Read the model definition and answer for the solid it produces. Units are mm, in the model's axes. Face numbers are marked on the shaded views. A direction names the side the tool comes from. Coordinates: 2 decimals unless noted, no trailing zeros. Write each loop counter-clockwise with the first axis right and the second up, starting at its lowest first coordinate (ties: lowest second). Pieces come first, ordered by that corner, then holes.
(1) Given pin 1 (1.5 mm diameter, centred on x = -4.5, y = 2, fed in from +Z); pin 2 (10.5 mm diameter, centred on x = 0, y = -3, fed in from +Z); pin 3 (1.5 mm diameter, centred on y = 7.5, z = 14.5, fed in from -X); pin 4 (3.5 mm diameter, centred on x = 0, y = 0, fed in from +Z), each flat-ended and moving along its own axis, determine where each tip first touches the part or whether it passes through.
(2) Which of the six approach directions +Z, -Z, +X, -X, +Y, -Y give full straight-line access (tool end or side, diameter ignored) to the marked faces 4 and 5?
(3) Find the intervals of material crossed by probe 1 along Y at (x, z) = (0, 3.55) (3 decimals); probe 2 along Y at (x, z) = (0, 8.45) (3 decimals); probe 3 along Z at (x, y) = (-6, 1.5), in increasing order.
(4) The mould has two halves that part along X. Classify the marked faces 1, 2 and 3: +X half, -X half, draft (parallel to the pull), parting line (faces both ways), or undercut.
(5) Section D-D on z = 10.5 is taken. Write down the section's boundary in (x, y) (3 decimals).
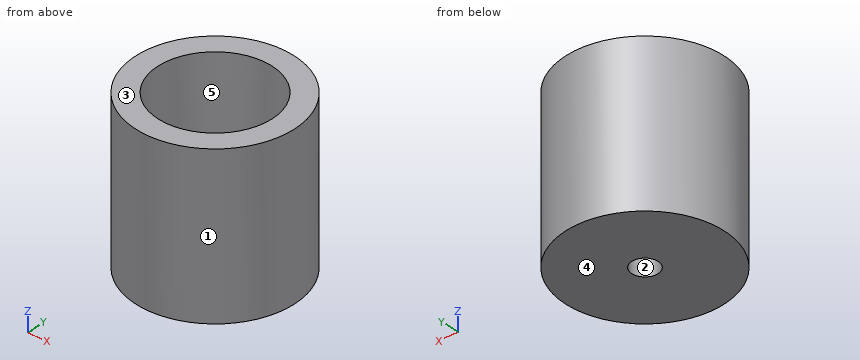
from build123d import *

# Parameters (mm, degrees)
SKETCH1_R                                        = 9.525
BOSS_EXTRUDE1_DEPTH                              = 19.05
CBORE_FOR_1_4_SOCKET_HEAD_CAP_SCREW1_D           = 0.79375
CBORE_FOR_1_4_SOCKET_HEAD_CAP_SCREW1_DEPTH       = 12.7
CBORE_FOR_1_4_SOCKET_HEAD_CAP_SCREW1_CBORE_D     = 3.175
CBORE_FOR_1_4_SOCKET_HEAD_CAP_SCREW1_CBORE_DEPTH = 3.175
CBORE_FOR_1_4_SOCKET_HEAD_CAP_SCREW1_TIP         = 0.238466558


with BuildPart() as part:
    # Sketch1 → Boss-Extrude1 (new body)
    with BuildSketch(Plane.XY):
        Circle(SKETCH1_R)
    extrude(amount=BOSS_EXTRUDE1_DEPTH)

    # Sketch6 → 1/4 NPT Tapped Hole1 (revolve, cut)
    with BuildSketch(Plane(origin=(0, 0, 19.05), x_dir=(0, -1, 0), z_dir=(1, 0, 0))):
        Polygon((0, 0), (0, 14.772347279), (5.5626, 11.43), (5.5626, 10.0203), (6.557978799, 10.0203), (6.858, 0), align=None)
    revolve(axis=Axis((0, 0, 25.4), (0, 0, -1)), mode=Mode.SUBTRACT)

    # CBORE for 1/4 Socket Head Cap Screw1
    with Locations(Plane(origin=(0, 0, 0), x_dir=(-1, 0, 0), z_dir=(0, 0, -1))):
        with Locations((0, 0)):
            CounterBoreHole(CBORE_FOR_1_4_SOCKET_HEAD_CAP_SCREW1_D / 2, CBORE_FOR_1_4_SOCKET_HEAD_CAP_SCREW1_CBORE_D / 2, CBORE_FOR_1_4_SOCKET_HEAD_CAP_SCREW1_CBORE_DEPTH, depth=CBORE_FOR_1_4_SOCKET_HEAD_CAP_SCREW1_DEPTH)
            with Locations((0, 0, -(CBORE_FOR_1_4_SOCKET_HEAD_CAP_SCREW1_DEPTH + CBORE_FOR_1_4_SOCKET_HEAD_CAP_SCREW1_TIP / 2))):  # 118° drill point
                Cone(0, CBORE_FOR_1_4_SOCKET_HEAD_CAP_SCREW1_D / 2, CBORE_FOR_1_4_SOCKET_HEAD_CAP_SCREW1_TIP, mode=Mode.SUBTRACT)


solid = part.part
Response:
1. pin 1: stops at z = 9.03
1. pin 2: stops at z = 19.05
1. pin 3: stops at x = -6.72
1. pin 4: stops at z = 5.33
2. face 4: -Z, +X, -X, +Y, -Y
2. face 5: +Z
3. probe 1: y = -9.525 to -0.397, 0.397 to 9.525
3. probe 2: y = -9.525 to -5.563, 5.563 to 9.525
3. probe 3: z = 0 to 9.03
4. face 1: parting line
4. face 2: undercut
4. face 3: draft
5. outline: circle Ø19.05 at (0, 0); hole circle Ø13.204 at (0, 0)
